```python
from build123d import *

# Parameters (mm, degrees)
SKETCH_1_W          = 25
SKETCH_1_H          = 41
EXTRUDE_1_DEPTH     = 50
FILLET_1_R          = 1
SKETCH_2_R          = 24.95
CUT_EXTRUDE_3_DEPTH = 41
FILLET_2_R          = 1


with BuildPart() as part:
    # Эскиз1 → Бобышка-Вытянуть1 (new body)
    with BuildSketch(Plane(origin=(0, 0, 0), x_dir=(1, 0, 0), z_dir=(0, 1, 0))):
        Rectangle(SKETCH_1_W, SKETCH_1_H)
    extrude(amount=EXTRUDE_1_DEPTH)

    # Скругление1
    fillet_1_edges = [part.edges().sort_by_distance(p)[0] for p in [
        (-12.5, 0, 0),
    ]]
    fillet(fillet_1_edges, radius=FILLET_1_R)

    # Эскиз2 → Вырез-Вытянуть3 (cut)
    with BuildSketch(Plane.XY.offset(20.5)):
        with Locations((12.5, 25)):
            Circle(SKETCH_2_R)
    extrude(amount=-CUT_EXTRUDE_3_DEPTH, mode=Mode.SUBTRACT)

    # Скругление2
    fillet_2_edges = [part.edges().sort_by_distance(p)[0] for p in [
        (-12.5, 50, 0),
    ]]
    fillet(fillet_2_edges, radius=FILLET_2_R)


solid = part.part
```
Work out the finished part from the listing and answer in its coordinate system (mm). Give positions to 0.01 mm unless a question says otherwise; leave off trailing zeros. Write each loop counter-clockwise with the first axis right and the second up, starting at its lowest first coordinate (ties: lowest second). Pieces come first, ordered by that corner, then holes. Notation, with made-up numbers: (55.25, 24) - (78.25, 24) arc R18 ccw to (78.25, 30) - close; hole circle Ø7 at (-39.5, 15.5). An arc over 180 degrees is marked (long way). Use one line per item in the form item = value.
1. A cutting plane is placed at B-B (z = -16). Write down the section's boundary in (x, y), and give its area (3 significant figures).
Filled in:
outline = (-12.5, 1) arc R1 ccw to (-11.5, 0) - (12.5, 0) - (12.5, 0.05) arc R24.95 cw to (12.5, 49.95) - (12.5, 50) - (-11.5, 50) arc R1 ccw to (-12.5, 49) - close
area = 272 mm^2
2. A cutting plane is placed at A-A (x = 1). Write down the section's boundary in (y, z), and give its area (3 significant figures).
Filled in:
outline = (0, -20.5) - (2.86, -20.5) - (2.86, 20.5) - (0, 20.5) - close; (47.14, -20.5) - (50, -20.5) - (50, 20.5) - (47.14, 20.5) - close
area = 234 mm^2
3. Each of these flat-tipped pins is pushed along its axis until it touches: pin 1 Ø10 at (y, z) = (20, -10) entering from +X; pin 2 Ø4 at (y, z) = (27, -2) entering from +X. Where does it stop, or does it pass through?
Filled in:
pin_1 = -10.36
pin_2 = -12.13
4. Determine the mould class of faces 1 (the face through (0, 50, 0)), 2 (the face through (-12.1, 30.4, -20.5)), 3 (the face through (-11.127, 16.984, 0.287)) for opening direction Y: released by +Y, released by -Y, zero draft, split by the parting line, or undercut.
Filled in:
face_1 = released by +Y
face_2 = zero draft
face_3 = undercut
5. Consider L1, parallel to Y at x = 7.25, z = -3; L2, parallel to Y at x = 4.25, z = -15.5; L3, parallel to X at y = 19.5, z = -1.5. Determine where each line is inside the solid, lowest interval first.
Filled in:
L1 = 0 to 0.61, 49.39 to 50
L2 = 0 to 1.45, 48.55 to 50
L3 = -12.5 to -11.84
6. A cutting plane is placed at C-C (x = -6). Write down the section's boundary in (y, z).
Filled in:
outline = (0, -20.5) - (8.26, -20.5) - (8.26, 20.5) - (0, 20.5) - close; (41.74, -20.5) - (50, -20.5) - (50, 20.5) - (41.74, 20.5) - close
